Could you check a few things on this model? Use its own coordinates, in mm. Give positions to 0.01 mm unless a question says otherwise; leave off trailing zeros. Loops run counter-clockwise (first coordinate to the right, second up) from the corner with the lowest first, then second, coordinate; pieces in that order, holes last. Notation, with made-up numbers: (7, 65.5) - (64, 65.5) arc R7 ccw to (64, 69.5) - close; hole circle Ø9 at (30, 49). An arc over 180 degrees is marked (long way). Answer in a Markdown table with one row per item. Add a question column.
```python
from build123d import *

# Parameters (mm, degrees)
SKETCH1_W                               = 635
SKETCH1_H                               = 150
BASE_EXTRUDE_DEPTH                      = 10
SKETCH2_W                               = 5
SKETCH2_H                               = 5
CUT_EXTRUDE1_DEPTH                      = 641.097648801
M5_0_5_000000_DIAMETER_HOLE1_AT_2_COUNT = 2
M5_0_5_000000_DIAMETER_HOLE1_AT_2_PITCH = 110


with BuildPart() as part:
    # Sketch1 → Base-Extrude (new body)
    with BuildSketch(Plane.XY):
        with Locations((0, 5)):
            Rectangle(SKETCH1_W, SKETCH1_H)
    extrude(amount=BASE_EXTRUDE_DEPTH)

    # Sketch2 → Cut-Extrude1 (cut, through all)
    with BuildSketch(Plane(origin=(317.5, 0, 0), x_dir=(0, 0, -1), z_dir=(1, 0, 0))):
        with Locations((-7.5, -57.5)):
            Rectangle(SKETCH2_W, SKETCH2_H)
    extrude(amount=-CUT_EXTRUDE1_DEPTH, mode=Mode.SUBTRACT)

    # Sketch4 → M5.0 (5.000000) Diameter Hole1 (revolve, cut)
    with BuildSketch(Plane(origin=(317.5, 70, 5), x_dir=(0, 0, -1), z_dir=(0, 1, 0))):
        Polygon((0, 0), (0, 16.502151548), (2.5, 15), (2.5, 0), align=None)
    m5_0_5_000000_diameter_hole1 = revolve(axis=Axis((323.85, 70, 5), (-1, 0, 0)), mode=Mode.SUBTRACT)

    # M5.0 (5.000000) Diameter Hole1 at 2: M5.0 (5.000000) Diameter Hole1 ×2
    with Locations(*[(0, -i * M5_0_5_000000_DIAMETER_HOLE1_AT_2_PITCH, 0) for i in range(1, M5_0_5_000000_DIAMETER_HOLE1_AT_2_COUNT)]):
        add(m5_0_5_000000_diameter_hole1, mode=Mode.SUBTRACT)

    # Mirror1: M5.0 (5.000000) Diameter Hole1 across plane
    add(m5_0_5_000000_diameter_hole1.mirror(Plane(origin=(0, 0, 0), x_dir=(0, 0, 1), z_dir=(1, 0, 0))), mode=Mode.SUBTRACT)

    # Mirror1 copy 1 sketch → Mirror1 copy 1 (revolve, cut)
    with BuildSketch(Plane(origin=(-317.5, -40, 5), x_dir=(0, 0, -1), z_dir=(0, 1, 0))):
        Polygon((0, 0), (0, -16.502151548), (2.5, -15), (2.5, 0), align=None)
    revolve(axis=Axis((-323.85, -40, 5), (-1, 0, 0)), mode=Mode.SUBTRACT)


solid = part.part
```
(1) I want a section at A-A on x = -85.5. Please give me the cut outline in (y, z), then the cut area to 4 significant figures.
(2) Please list where these lines run through material, in increasing order: line 1 (Y direction, x = -144.5, z = 9); line 2 (Z direction, x = 314.25, y = -40).
(3) For pin 1 Ø4.5 at (y, z) = (70, 5) entering from +X; pin 2 Ø6 at (y, z) = (70, 5) entering from +X; pin 3 Ø2.5 at (x, y) = (114, -57) entering from +Z, each with a flat end and sliding along its axis, tell me the tip position at first contact or that it passes through.
Reported:
| question | item | result |
|---|---|---|
| 1 | outline | (-70, 0) - (80, 0) - (80, 10) - (-55, 10) - (-55, 5) - (-60, 5) - (-60, 10) - (-70, 10) - close |
| 1 | area | 1,475 mm² |
| 2 | line 1 | -70 to -60, -55 to 80 |
| 2 | line 2 | 0 to 2.5, 7.5 to 10 |
| 3 | pin 1 | x = 302.35 |
| 3 | pin 2 | x = 317.5 |
| 3 | pin 3 | z = 5 |
